```python
from build123d import *

# Parameters (mm, degrees)
BOSS_EXTRUDE1_DEPTH = 2
CUT_EXTRUDE1_DEPTH  = 15.560219779
CUT_EXTRUDE2_DEPTH  = 1.5
FILLET1_R           = 0.5


with BuildPart() as part:
    # Sketch1 → Boss-Extrude1 (new body)
    with BuildSketch(Plane.XY):
        Polygon((0, 8), (8, 0), (0, 0), (-12, 0), (-12, 8), align=None)
    extrude(amount=BOSS_EXTRUDE1_DEPTH)

    # Sketch2 → Cut-Extrude1 (cut, through all)
    with BuildSketch(Plane.XY.offset(2)):
        Polygon((-0.621320344, 6.5), (4.378679656, 1.5), (-0.621320344, 1.5), (-10.5, 1.5), (-10.5, 6.5), align=None)
    extrude(amount=-CUT_EXTRUDE1_DEPTH, mode=Mode.SUBTRACT)

    # Sketch3 → Cut-Extrude2 (cut)
    with BuildSketch(Plane(origin=(0, 0, 0), x_dir=(-1, 0, 0), z_dir=(0, 0, -1))):
        Polygon((0.414213562, 7), (-5.585786438, 1), (0.414213562, 1), (11, 1), (11, 7), align=None)
    extrude(amount=-CUT_EXTRUDE2_DEPTH, mode=Mode.SUBTRACT)

    # Fillet1
    fillet1_edges = [part.edges().sort_by_distance(p)[0] for p in [
        (4.378679656, 1.5, 1.75),
        (-10.5, 1.5, 1.75),
        (-0.621320344, 6.5, 1.75),
        (-10.5, 6.5, 1.75),
    ]]
    fillet(fillet1_edges, radius=FILLET1_R)


solid = part.part
```
Verification items for the finished model (mm, model axes). A direction names the side the tool comes from. Coordinates: 2 decimals unless noted, no trailing zeros. Loops run counter-clockwise (first coordinate to the right, second up) from the corner with the lowest first, then second, coordinate; pieces in that order, holes last. Notation, with made-up numbers: (81, -23.75) -> (99, -23.75) arc R34 cw to (99, 7.25) -> close; hole circle Ø5 at (0, -5.5). An arc over 180 degrees is marked (long way). Answer in a Markdown table with one row per item. Add a question column.
1. Draft check along Y on faces 1 (the face through (-6, 7, 1)), 2 (the face through (-2, 0, 1)), 3 (the face through (-6, 8, 1)). Enter one of: +Y half, -Y half, draft (parallel to the pull), parting line (faces both ways), or undercut.
2. Section check C-C, the plane y = 4. Enter the section's corners in (x, z).
3. Material ranges on probe 1 along Y at (x, z) = (-7, 0.7); probe 2 along Y at (x, z) = (-9.75, 1.55); probe 3 along X at (y, z) = (5, 1.1), recorded low to high. Write a range as [from, to].
4. Section check A-A, the plane x = -6.25. Enter the section's corners in (y, z), then the cut area to 3 significant figures.
5. Section check D-D, the plane x = 4. Enter the section's corners in (y, z).
6. Section check B-B, the plane z = 0.9. Enter the section's corners in (x, y).
7. Access from +Z, -Z, +X, -X, +Y, -Y to the whole of each face (thin tool, end or side, straight path). Record for faces 4 (the face through (-11, 4, 1)), 5 (the face through (1.5, 4.38, 1.75)), 6 (the face through (-12, 4, 1)).
8. Depth check by flat-ended pin: P1, Ø0.8, axis at y = 4.5, z = 1, coming from the +X side; P2, Ø2, axis at x = 5.5, y = 5.5, coming from the +Z side. Enter the tip coordinate at first touch or a pass-through.
Derived:
| question | item | result |
|---|---|---|
| 1 | face 1 | undercut |
| 1 | face 2 | -Y half |
| 1 | face 3 | +Y half |
| 2 | outline | (-12, 0) -> (-11, 0) -> (-11, 1.5) -> (-10.5, 1.5) -> (-10.5, 2) -> (-12, 2) -> close; (1.88, 1.5) -> (2.59, 1.5) -> (2.59, 0) -> (4, 0) -> (4, 2) -> (1.88, 2) -> close |
| 3 | probe 1 | y = [0, 1], [7, 8] |
| 3 | probe 2 | y = [0, 1.5], [6.5, 8] |
| 3 | probe 3 | x = [-12, -11], [1.59, 3] |
| 4 | outline | (0, 0) -> (1, 0) -> (1, 1.5) -> (1.5, 1.5) -> (1.5, 2) -> (0, 2) -> close; (6.5, 1.5) -> (7, 1.5) -> (7, 0) -> (8, 0) -> (8, 2) -> (6.5, 2) -> close |
| 4 | area | 4.50 mm² |
| 5 | outline | (0, 0) -> (1, 0) -> (1, 1.5) -> (2.59, 1.5) -> (2.59, 0) -> (4, 0) -> (4, 2) -> (0, 2) -> close |
| 6 | outline | (-12, 0) -> (8, 0) -> (0, 8) -> (-12, 8) -> close; hole (-11, 1) -> (5.59, 1) -> (-0.41, 7) -> (-11, 7) -> close |
| 7 | face 4 | -Z |
| 7 | face 5 | +Z, -Z |
| 7 | face 6 | +Z, -Z, -X, +Y, -Y |
| 8 | P1 | stops at x = 3.9 |
| 8 | P2 | passes through |
